Here's how the part is built. I have some questions about the finished solid (model axes, mm). Give positions to 0.01 mm unless a question says otherwise; leave off trailing zeros. Loops run counter-clockwise (first coordinate to the right, second up) from the corner with the lowest first, then second, coordinate; pieces in that order, holes last. Notation, with made-up numbers: M 66,58.25 L 105,58.25 A26 cw 105,83.25 Z; hole C -33.75,88.5 d6. An arc over 180 degrees is marked long. Answer as CSV lines item,"result". Start each with the question number.
Item 1: Will these pins go through, and if not, where does the flat tip stop? P1, Ø1.5, axis at x = 8.5, z = 2, coming from the -Y side; P2, Ø0.8, axis at x = -1, z = 1.5, coming from the -Y side.
Item 2: If I drill on line 1 along Y through (x, z) = (0, 1.3); line 2 along Y through (x, z) = (-6, 1.7); line 3 along X through (y, z) = (-5.5, 0.7), over which ranges is the centre line in solid material (lowest first)? Write a range as from..to.
Item 3: I want a section at D-D on z = 0.6. Give the number of separate pieces and of enclosed holes in the cut face, plus the area to 3 significant figures.
Item 4: I want a section at C-C on y = -8.75. List the corners of the cut face in (x, z) for me, plus the area to 3 significant figures.
Item 5: If we mould it in two halves opening along X, with no side actions, what happens to faces 1 (the flat face through (0.3, -10, 1.4)), 2 (the flat face through (0, -3, 2.8))? For each: released by +X, released by -X, zero draft, split by the parting line, or undercut.
Item 6: I want a section at B-B on y = 1.5. List the corners of the cut face in (x, z) for me.
Item 7: I want a section at A-A on x = -10.5. List the corners of the cut face in (y, z) for me, plus the area to 3 significant figures.
from build123d import *

# Parameters (mm, degrees)
SKETCH_R           = 12.9
PAD_DEPTH          = 2.8
POCKET_DEPTH       = 2.801
POCKET001_DEPTH    = 75.988977
POLARPATTERN_COUNT = 20


with BuildPart() as part:
    # Sketch → Pad (new body)
    with BuildSketch(Plane.XY):
        Circle(SKETCH_R)
    extrude(amount=PAD_DEPTH)

    # Sketch001 → Pocket (cut, through all)
    with BuildSketch(Plane.XY.offset(2.8)):
        with BuildLine():
            ThreePointArc((-3.5, 2), (-5.5, 0), (-3.5, -2))
            Line((-3.5, -2), (3.5, -2))
            ThreePointArc((3.5, -2), (5.5, 0), (3.5, 2))
            Line((-3.5, 2), (3.5, 2))
        make_face()
    extrude(amount=-POCKET_DEPTH, mode=Mode.SUBTRACT)

    # Sketch002 → Pocket001 (cut, through all)
    with BuildSketch(Plane.XY.offset(2.8)):
        Polygon((-0.5, 11.979325), (0.5, 11.979325), (0.1, 7.999375), (-0.1, 7.999375), align=None)
    pocket001 = extrude(amount=-POCKET001_DEPTH, mode=Mode.SUBTRACT)

    # PolarPattern: Pocket001 ×20 about axis
    polarpattern_axis = Axis((0, 0, 2.8), (0, 0, 1))
    for i in range(1, POLARPATTERN_COUNT):
        add(pocket001.rotate(polarpattern_axis, i * 360 / POLARPATTERN_COUNT), mode=Mode.SUBTRACT)


solid = part.part
Result:
1,P1,"y = -10.31"
1,P2,"y = -12.89"
2,line 1,"-12.9..-11.98, -8..-2, 2..8, 11.98..12.9"
2,line 2,"-11.42..-8.89, -7.78..7.78, 8.89..11.42"
2,line 3,"-11.67..-8.04, -7.22..7.22, 8.04..11.67"
3,separate pieces,"1"
3,enclosed holes,"21"
3,area,"434 mm^2"
4,outline,"M -9.48,0 L -6.87,0 L -6.87,2.8 L -9.48,2.8 Z; M -5.92,0 L -3.08,0 L -3.08,2.8 L -5.92,2.8 Z; M -2.62,0 L -0.18,0 L -0.18,2.8 L -2.62,2.8 Z; M 0.18,0 L 2.62,0 L 2.62,2.8 L 0.18,2.8 Z; M 3.08,0 L 5.92,0 L 5.92,2.8 L 3.08,2.8 Z; M 6.87,0 L 9.48,0 L 9.48,2.8 L 6.87,2.8 Z"
4,area,"44.2 mm^2"
5,face 1,"undercut"
5,face 2,"zero draft"
6,outline,"M -12.81,0 L -4.82,0 L -4.82,2.8 L -12.81,2.8 Z; M 4.82,0 L 12.81,0 L 12.81,2.8 L 4.82,2.8 Z"
7,outline,"M -7.49,0 L -3.85,0 L -3.85,2.8 L -7.49,2.8 Z; M -3,0 L -0.35,0 L -0.35,2.8 L -3,2.8 Z; M 0.35,0 L 3,0 L 3,2.8 L 0.35,2.8 Z; M 3.85,0 L 7.49,0 L 7.49,2.8 L 3.85,2.8 Z"
7,area,"35.2 mm^2"
